Can you work these out from the model? Positions are in its coordinate system, mm. Face numbers are marked on the shaded views. A direction names the side the tool comes from. Give positions to 0.01 mm unless a question says otherwise; leave off trailing zeros. Order: outer loops, then holes, each group sorted by start corner. A loop starts at its lowest first (then second) coordinate and runs counter-clockwise, first axis right, second up. Notation, with made-up numbers: (-27.5, -13) - (25.5, -13) arc R13 cw to (25.5, 9) - close; hole circle Ø9 at (-9.75, 13.25). An arc over 180 degrees is marked (long way). Use one line per item in the form item = value. Start each with the question number.
1) Which directions (+Z, -Z, +X, -X, +Y, -Y) give clear straight access to the entire face, cutting with the end or side of a thin tool? Please do the marked faces 1, 2 and 3.
2) We'd pull the mould along Z, two halves only. Please class the marked faces 4, 5, 6 and 7: released by +Z, released by -Z, zero draft, split by the parting line, or undercut.
3) Suppose I cut it at D-D, the plane z = 10. Write out the boundary of the cut face in (x, y), and give its area (3 significant figures).
4) Suppose I cut it at A-A, the plane z = -1.75. Write out the boundary of the cut face in (x, y), and give its area (3 significant figures).
5) Suppose I cut it at B-B, the plane y = 11. Write out the boundary of the cut face in (x, z), and give its area (3 significant figures).
6) Suppose I cut it at C-C, the plane x = -1. Write out the boundary of the cut face in (y, z), and give its area (3 significant figures).
7) Please list where these lines run through material, in increasing order: probe 1 along Y at (x, z) = (-18.5, -6.25); probe 2 along Y at (x, z) = (-16, -3.25); probe 3 along Y at (x, z) = (-13, -6.5).
8) For pin 1 (10 mm diameter, centred on x = -2.5, z = 1, fed in from +Y); pin 2 (6 mm diameter, centred on y = 13.5, z = 12.5, fed in from +X), each with a flat end and sliding along its axis, tell me the tip position at first contact or that it passes through.
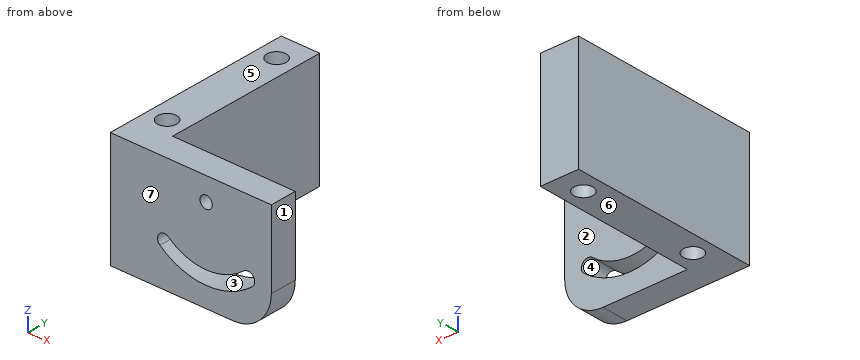
```python
from build123d import *

# Parameters (mm, degrees)
SKETCH1_W           = 10
SKETCH1_H           = 30
SKETCH1_R           = 1.6
BOSS_EXTRUDE1_DEPTH = 7
SKETCH1_3_W         = 10
SKETCH1_3_H         = 30
BOSS_EXTRUDE2_DEPTH = 50
SKETCH2_R           = 2.5
CUT_EXTRUDE1_DEPTH  = 63.790013573


with BuildPart() as part:
    # Sketch1 → Boss-Extrude1 (new body)
    # profile 1 of 2: a face of its own
    with BuildSketch(Plane(origin=(0, 0, 0), x_dir=(1, 0, 0), z_dir=(0, 1, 0))):
        with Locations((-18.293471286, -6.131670173)):
            Rectangle(SKETCH1_W, SKETCH1_H)
    # profile 2 of 2: a face of its own
    with BuildSketch(Plane(origin=(0, 0, 0), x_dir=(1, 0, 0), z_dir=(0, 1, 0))):
        with BuildLine():
            Line((1.706528714, 8.868329827), (-13.293471286, 8.868329827))
            Line((-13.293471286, 8.868329827), (-13.293471286, -21.131670173))
            Line((-13.293471286, -21.131670173), (1.706528714, -21.131670173))
            Line((1.706528714, -21.131670173), (18.706528714, -21.131670173))
            Line((18.706528714, -21.131670173), (18.706528714, -1.131670173))
            ThreePointArc((18.706528714, -1.131670173), (15.777596526, 5.939397639), (8.706528714, 8.868329827))
            Line((8.706528714, 8.868329827), (1.706528714, 8.868329827))
        make_face()
        with Locations(Location((1.706528714, -15.131670173, 0), (0, 0, 270))):
            Circle(SKETCH1_R, mode=Mode.SUBTRACT)
        with BuildLine():
            ThreePointArc((-10.345738968, -0.768336864), (1.706528714, 3.618329827), (13.758796396, -0.768336864))
            ThreePointArc((13.758796396, -0.768336864), (13.974495854, -3.233792957), (11.509039762, -3.449492415))
            ThreePointArc((11.509039762, -3.449492415), (1.706528714, 0.118329827), (-8.095982334, -3.449492415))
            ThreePointArc((-8.095982334, -3.449492415), (-10.561438426, -3.233792957), (-10.345738968, -0.768336864))
        make_face(mode=Mode.SUBTRACT)
    extrude(amount=BOSS_EXTRUDE1_DEPTH)

    # Sketch1_3 → Boss-Extrude2 (add)
    with BuildSketch(Plane(origin=(0, 0, 0), x_dir=(1, 0, 0), z_dir=(0, 1, 0))):
        with Locations((-18.293471286, -6.131670173)):
            Rectangle(SKETCH1_3_W, SKETCH1_3_H)
    extrude(amount=BOSS_EXTRUDE2_DEPTH)

    # Sketch2 → Cut-Extrude1 (cut, through all)
    with BuildSketch(Plane(origin=(0, 0, -8.868329827), x_dir=(-1, 0, 0), z_dir=(0, 0, -1))):
        with Locations((18.293471286, 43)):
            Circle(SKETCH2_R)
        with Locations((18.293471286, 11)):
            Circle(SKETCH2_R)
    extrude(amount=-CUT_EXTRUDE1_DEPTH, mode=Mode.SUBTRACT)


solid = part.part
```
Result sheet:
q1.face_1 = +Z, -Z, +X, +Y, -Y
q1.face_2 = +Z, -Z, +X, +Y
q1.face_3 = +Y, -Y
q2.face_4 = undercut
q2.face_5 = released by +Z
q2.face_6 = released by -Z
q2.face_7 = zero draft
q3.outline = (-23.29, 0) - (18.71, 0) - (18.71, 7) - (-13.29, 7) - (-13.29, 50) - (-23.29, 50) - close; hole circle Ø5 at (-18.29, 11); hole circle Ø5 at (-18.29, 43)
q3.area = 685 mm²
q4.outline = (-23.29, 0) - (-6.45, 0) - (-6.45, 7) - (-13.29, 7) - (-13.29, 50) - (-23.29, 50) - close; (9.87, 0) - (18.28, 0) - (18.28, 7) - (9.87, 7) - close; hole circle Ø5 at (-18.29, 11); hole circle Ø5 at (-18.29, 43)
q4.area = 568 mm²
q5.outline = (-23.29, -8.87) - (-20.79, -8.87) - (-20.79, 21.13) - (-23.29, 21.13) - close; (-15.79, -8.87) - (-13.29, -8.87) - (-13.29, 21.13) - (-15.79, 21.13) - close
q5.area = 150 mm²
q6.outline = (0, -8.87) - (7, -8.87) - (7, -3.42) - (0, -3.42) - close; (0, 0.12) - (7, 0.12) - (7, 21.13) - (0, 21.13) - close
q6.area = 185 mm²
q7.probe_1 = 0 to 8.51, 13.49 to 40.51, 45.49 to 50
q7.probe_2 = 0 to 10.01, 11.99 to 42.01, 43.99 to 50
q7.probe_3 = 0 to 7
q8.pin_1 = 7
q8.pin_2 = -13.29
